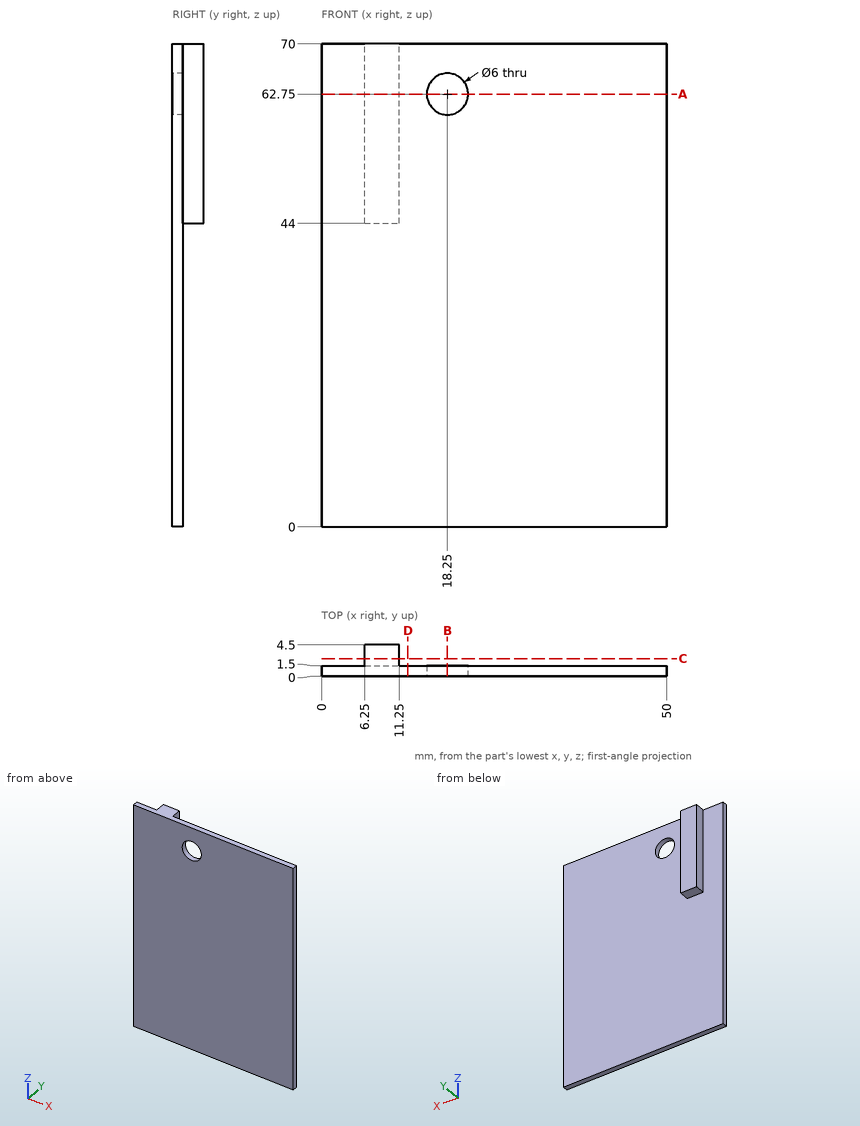
Part print with two shaded views. Sizes in mm from the minimum x, y, z corner. Round coordinates to 2 decimals unless told otherwise and drop trailing zeros. Order: outer loops, then holes, each group sorted by start corner. A loop starts at its lowest first (then second) coordinate and runs counter-clockwise, first axis right, second up. Notation, with made-up numbers: (-4, 55.5) - (10, 55.5) arc R16 cw to (10, 77.5) - close; hole circle Ø2 at (28.5, 24.25). An arc over 180 degrees is marked (long way). Answer as CSV lines item,"result". Start each with the question number.
1. Drill centre lines: L1, parallel to Z at x = 18.25, y = 0.8; L2, parallel to Z at x = 11, y = 4.25; L3, parallel to Y at x = 42.5, z = 7. Where is each one in solid material? Low to high. Write a range as [from, to].
2. Pin check, flat tips, straight feed: pin 1 (5.5 mm diameter, centred on x = 18.25, z = 62.75, fed in from -Y); pin 2 (8 mm diameter, centred on x = 38, z = 34, fed in from +Y); pin 3 (1.5 mm diameter, centred on y = 3.5, z = 56.5, fed in from +X); pin 4 (1.5 mm diameter, centred on y = 3.5, z = 58.5, fed in from -X). Stop position of each tip, or through.
3. Saw through at C-C, the plane y = 2.5. Write the cut outline in (x, z), and give its area (3 significant figures).
4. Saw through at D-D, the plane x = 12.5. Write the cut outline in (y, z).
5. Saw through at B-B, the plane x = 18.25. Write the cut outline in (y, z).
6. Saw through at A-A, the plane z = 62.75. Write the cut outline in (x, y).
Model answer:
1,L1,"z = [0, 59.75], [65.75, 70]"
1,L2,"z = [44, 70]"
1,L3,"y = [0, 1.5]"
2,pin 1,"passes through"
2,pin 2,"stops at y = 1.5"
2,pin 3,"stops at x = 11.25"
2,pin 4,"stops at x = 6.25"
3,outline,"(6.25, 44) - (11.25, 44) - (11.25, 70) - (6.25, 70) - close"
3,area,"130 mm²"
4,outline,"(0, 0) - (1.5, 0) - (1.5, 70) - (0, 70) - close"
5,outline,"(0, 0) - (1.5, 0) - (1.5, 59.75) - (0, 59.75) - close; (0, 65.75) - (1.5, 65.75) - (1.5, 70) - (0, 70) - close"
6,outline,"(0, 0) - (15.25, 0) - (15.25, 1.5) - (11.25, 1.5) - (11.25, 4.5) - (6.25, 4.5) - (6.25, 1.5) - (0, 1.5) - close; (21.25, 0) - (50, 0) - (50, 1.5) - (21.25, 1.5) - close"
